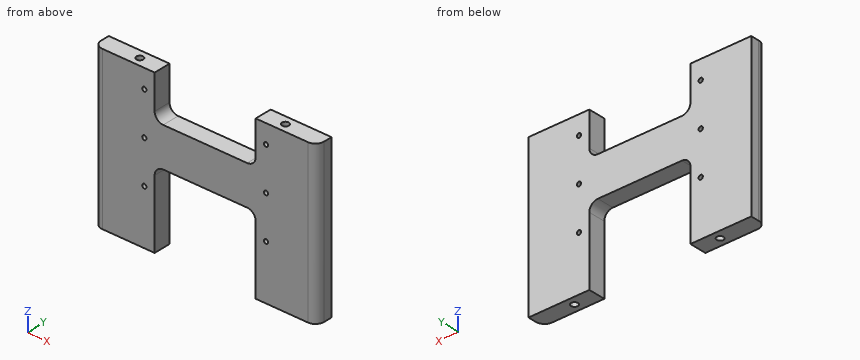
```python
from build123d import *

# Parameters (mm, degrees)
F0_R           = 1.25
F1_DEPTH       = 10
F2_R           = 5
F5_D           = 4
F5_DEPTH       = 15
F5_TIP         = 1.2017212381
F5_ON_F4_D     = 4
F5_ON_F4_DEPTH = 15
F5_ON_F4_TIP   = 1.2017212381


with BuildPart() as f1:
    # F0 (on Front) → F1 (new body)
    with BuildSketch(Plane.XZ):
        Polygon((-65, 43.3330013267), (-65, -49.6669986733), (-29.5, -49.6669986733), (-29.5, -4.6669986733), (0, -4.6669986733), (0, 18.3330013267), (-29.5, 18.3330013267), (-29.5, 43.3330013267), align=None)
        with Locations((-35.5, -42.6669986733)):
            Circle(F0_R, mode=Mode.SUBTRACT)
        with Locations((-35.5, -17.6669986733)):
            Circle(F0_R, mode=Mode.SUBTRACT)
        with Locations((-35.5, 7.3330013267)):
            Circle(F0_R, mode=Mode.SUBTRACT)
        with Locations((-35.5, 32.3330013267)):
            Circle(F0_R, mode=Mode.SUBTRACT)
        with Locations((-35.5, -42.6669986733)):
            Circle(F0_R)
    extrude(amount=F1_DEPTH)

    # F2
    f2_edges = [f1.edges().sort_by_distance(p)[0] for p in [
        (-65, -10, -3.166999),
        (-29.5, -5, -4.666999),
        (-29.5, -5, 18.333001),
    ]]
    fillet(f2_edges, radius=F2_R)

    # F5
    with Locations(Plane.XY.offset(43.3330013267)):
        with Locations((-42.5, -5)):
            Hole(F5_D / 2, depth=F5_DEPTH)
            with Locations((0, 0, -(F5_DEPTH + F5_TIP / 2))):  # 118° drill point
                Cone(0, F5_D / 2, F5_TIP, mode=Mode.SUBTRACT)

    # F5 on F4
    with Locations(Plane(origin=(0, 0, -49.6669986733), x_dir=(1, 0, 0), z_dir=(0, 0, -1))):
        with Locations((-42.5, 5)):
            Hole(F5_ON_F4_D / 2, depth=F5_ON_F4_DEPTH)
            with Locations((0, 0, -(F5_ON_F4_DEPTH + F5_ON_F4_TIP / 2))):  # 118° drill point
                Cone(0, F5_ON_F4_D / 2, F5_ON_F4_TIP, mode=Mode.SUBTRACT)

    # F6: F1 across plane


with BuildPart() as f1_1:
    add(f1.part)
    add(f1.part.mirror(Plane.YZ))


solid = f1_1.part
```
Here's how the part is built. I have some questions about the finished solid (model axes, mm). Coordinates: 2 decimals unless noted, no trailing zeros. Order: outer loops, then holes, each group sorted by start corner. A loop starts at its lowest first (then second) coordinate and runs counter-clockwise, first axis right, second up. Notation, with made-up numbers: (20.5, -2) -> (76.5, -2) arc R11 ccw to (76.5, 3) -> close; hole circle Ø9 at (-22.75, 34.25). An arc over 180 degrees is marked (long way). Return JSON: item names as keys, results as strings.
1) If we section it at B-B on x = -19.5: List the corners of the cut face in (y, z) for me.
Conclusion:
{"outline": "(-10, -4.67) -> (0, -4.67) -> (0, 18.33) -> (-10, 18.33) -> close"}
2) I'm going to push flat-ended pins straight in: P1, Ø2, axis at x = -35.5, z = 7.33, coming from the +Y side; P2, Ø3, axis at x = 1.5, y = -5.5, coming from the -Z side; P3, Ø3.5, axis at x = -42.5, y = -5, coming from the +Z side; P4, Ø2.5, axis at x = -42.5, y = -5, coming from the -Z side. Where does each tip first touch, or does it pass through?
Conclusion:
{"P1": "passes through", "P2": "stops at z = -4.67", "P3": "stops at z = 28.18", "P4": "stops at z = -34.22"}
3) If we section it at A-A on z = -14.5: List the corners of the cut face in (x, y) for me.
Conclusion:
{"outline": "(-65, -5) arc R5 ccw to (-60, -10) -> (-29.5, -10) -> (-29.5, 0) -> (-65, 0) -> close; (29.5, -10) -> (60, -10) arc R5 ccw to (65, -5) -> (65, 0) -> (29.5, 0) -> close"}
4) If I drill on probe 1 along Z at (x, y) = (-35.5, -4); probe 2 along Y at (x, z) = (42.5, -44.25); probe 3 along X at (y, z) = (-3.5, -41), over which ranges is the centre line in solid material (lowest first)?
Conclusion:
{"probe 1": "z = -49.67 to -18.92, -16.42 to 6.08, 8.58 to 31.08, 33.58 to 43.33", "probe 2": "y = -10 to -7, -3 to 0", "probe 3": "x = -65 to -43.82, -41.18 to -29.5, 29.5 to 41.18, 43.82 to 65"}
